For this review, use the dimensioned drawing (mm, ordinates from the lowest corner) and the shaded views. Give positions to 0.01 mm unless a question says otherwise; leave off trailing zeros. Write each loop counter-clockwise with the first axis right and the second up, starting at its lowest first coordinate (ties: lowest second). Pieces come first, ordered by that corner, then holes. Notation, with made-up numbers: (84, 10) -> (132, 10) arc R19 ccw to (132, 31) -> close; hole circle Ø3 at (88, 28). An arc over 180 degrees is marked (long way). Return JSON: item names as keys, results as strings.
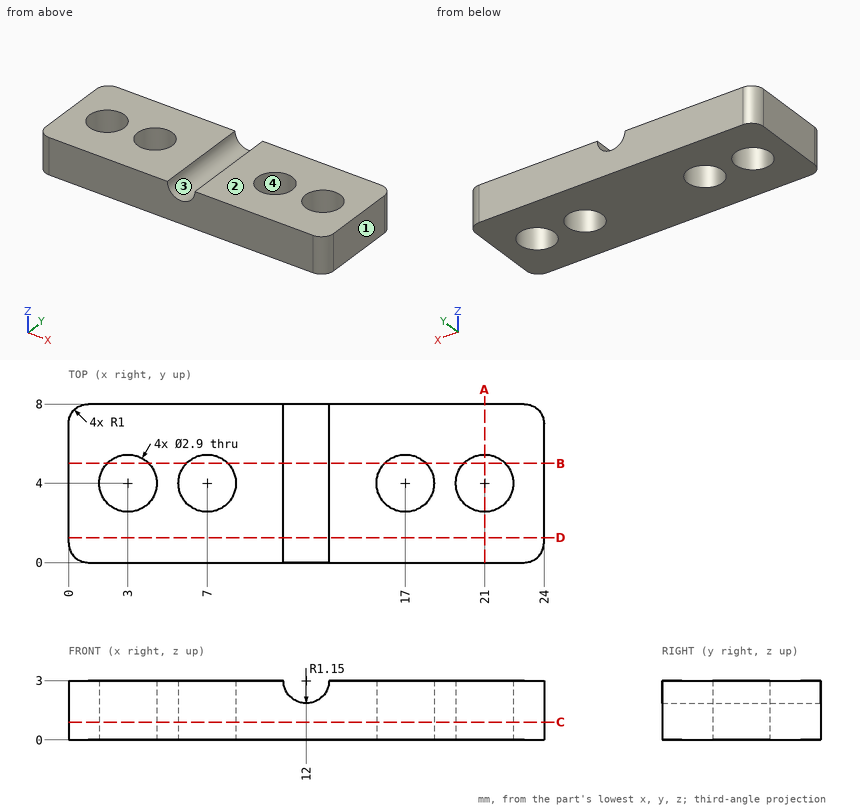
1. Add section C-C, the plane z = 0.9. State the section outline as (x, y) points, plus the area to 3 significant figures.
Results found:
{"outline": "(0, 1) arc R1 ccw to (1, 0) -> (23, 0) arc R1 ccw to (24, 1) -> (24, 7) arc R1 ccw to (23, 8) -> (1, 8) arc R1 ccw to (0, 7) -> close; hole circle Ø2.9 at (3, 4); hole circle Ø2.9 at (7, 4); hole circle Ø2.9 at (17, 4); hole circle Ø2.9 at (21, 4)", "area": "165 mm²"}
2. Add section A-A, the plane x = 21. State the section outline as (y, z) points.
Results found:
{"outline": "(0, 0) -> (2.55, 0) -> (2.55, 3) -> (0, 3) -> close; (5.45, 0) -> (8, 0) -> (8, 3) -> (5.45, 3) -> close"}
3. The part is to be moulded in two halves that separate along X. For the marked faces 1, 2, 3 and 4, say which applies: +X half, -X half, draft (parallel to the pull), parting line (faces both ways), or undercut.
Results found:
{"face 1": "+X half", "face 2": "draft", "face 3": "undercut", "face 4": "undercut"}
4. Add section D-D, the plane y = 1.25. State the section outline as (x, z) points.
Results found:
{"outline": "(0, 0) -> (24, 0) -> (24, 3) -> (13.15, 3) arc R1.15 cw to (10.85, 3) -> (0, 3) -> close"}
5. To check wall thickness, follow probe 1 along Y at (x, z) = (21, 1.15); probe 2 along X at (y, z) = (2.75, 2.8); probe 3 along X at (y, z) = (3.75, 0.35). State the ranges of each line that lie inside material, in increasing order.
Results found:
{"probe 1": "y = 0 to 2.55, 5.45 to 8", "probe 2": "x = 0 to 2.27, 3.73 to 6.27, 7.73 to 10.87, 13.13 to 16.27, 17.73 to 20.27, 21.73 to 24", "probe 3": "x = 0 to 1.57, 4.43 to 5.57, 8.43 to 15.57, 18.43 to 19.57, 22.43 to 24"}
6. Add section B-B, the plane y = 5. State the section outline as (x, z) points, plus the area to 3 significant figures.
Results found:
{"outline": "(0, 0) -> (1.95, 0) -> (1.95, 3) -> (0, 3) -> close; (4.05, 0) -> (5.95, 0) -> (5.95, 3) -> (4.05, 3) -> close; (8.05, 0) -> (15.95, 0) -> (15.95, 3) -> (13.15, 3) arc R1.15 cw to (10.85, 3) -> (8.05, 3) -> close; (18.05, 0) -> (19.95, 0) -> (19.95, 3) -> (18.05, 3) -> close; (22.05, 0) -> (24, 0) -> (24, 3) -> (22.05, 3) -> close", "area": "44.7 mm²"}
